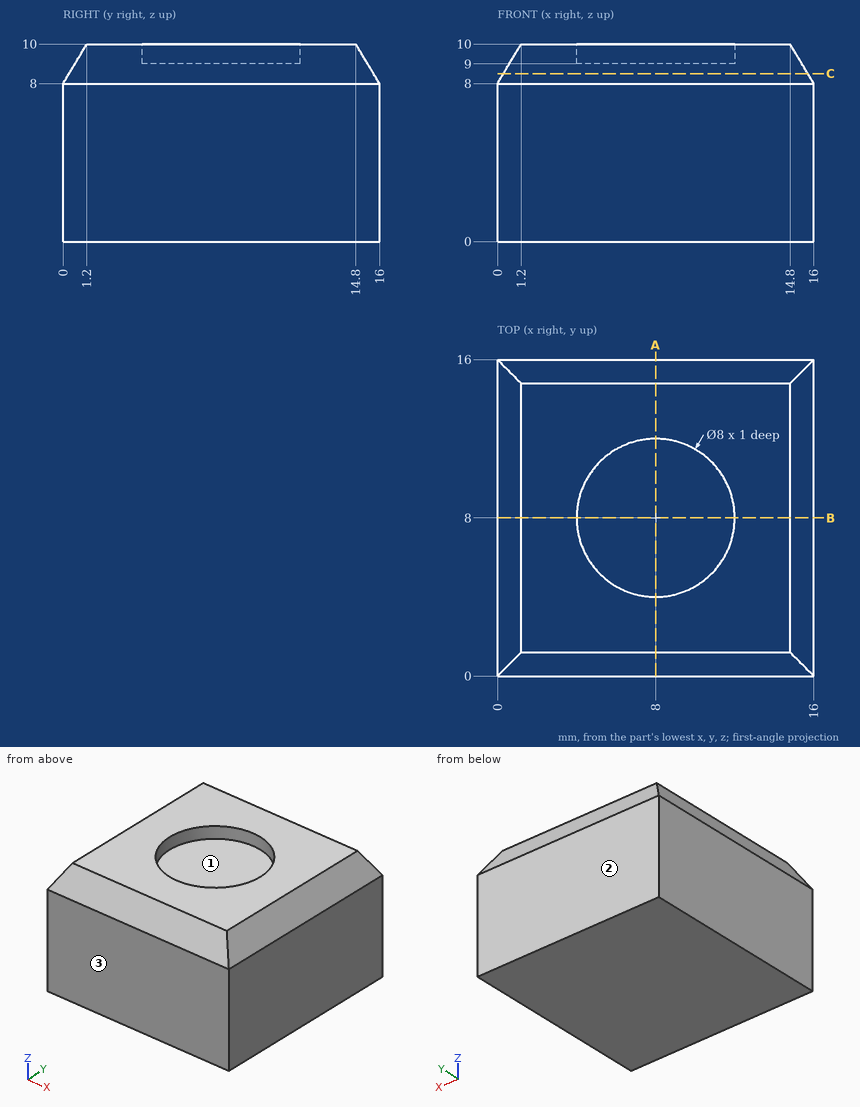
Check sheet for the drawn part. Datum: minimum x, y, z corner. Units: mm. Round coordinates to 2 decimals unless told otherwise and drop trailing zeros. Loops run counter-clockwise (first coordinate to the right, second up) from the corner with the lowest first, then second, coordinate; pieces in that order, holes last. Notation, with made-up numbers: (85.25, 49) - (121.25, 49) arc R25 cw to (121.25, 85) - close; hole circle Ø10 at (3, -17.5). An arc over 180 degrees is marked (long way). Write each question's results on one line, items separated by ' | '. Start each with the question number.
Q1. Gauge pin test, flat end, axial feed: P1, Ø7, axis at x = 8, y = 8, coming from the +Z side. Record the tip position at first contact, or that the pin passes through.
Q2. Thickness scan on line 1 (Y direction, x = 13.5, z = 9.25); line 2 (X direction, y = 7.5, z = 9.5); line 3 (Z direction, x = 1, y = 9). Record the ranges inside material, lowest first. Write a range as [from, to].
Q3. Cross-section at C-C on z = 8.5. Enter the section's corners in (x, y), and give its area (3 significant figures).
Q4. Release check for a two-part mould opening along Y. For the marked faces 1, 2 and 3 record: +Y half, -Y half, draft (parallel to the pull), parting line (faces both ways), or undercut.
Q5. Cross-section at A-A on x = 8. Enter the section's corners in (y, z).
Answers below:
1) P1: stops at z = 9
2) line 1: y = [0.75, 15.25] | line 2: x = [0.9, 4.03], [11.97, 15.1] | line 3: z = [0, 9.67]
3) outline: (0.3, 0.3) - (15.7, 0.3) - (15.7, 15.7) - (0.3, 15.7) - close | area: 237 mm²
4) face 1: undercut | face 2: +Y half | face 3: -Y half
5) outline: (0, 0) - (16, 0) - (16, 8) - (14.8, 10) - (12, 10) - (12, 9) - (4, 9) - (4, 10) - (1.2, 10) - (0, 8) - close
